Source: CAD feature listing. Evaluate the final solid. Frame: model axes, mm. A direction names the side the tool comes from. Round coordinates to 2 decimals unless told otherwise and drop trailing zeros. Write each loop counter-clockwise with the first axis right and the second up, starting at its lowest first coordinate (ties: lowest second). Pieces come first, ordered by that corner, then holes. Notation, with made-up numbers: M -21.5,50.5 L 32.5,50.5 A15 cw 32.5,74.5 Z; hole C 37,89.25 d4. An arc over 180 degrees is marked long. Use a Markdown table: item, result.
```python
from build123d import *

# Parameters (mm, degrees)
EXTRUDE_1_DEPTH          = 4
EXTRUDE_2_DEPTH          = 9
CHAMFER_1_SIZE           = 1
CHAMFER_2_SIZE           = 1
CHAMFER_3_SIZE           = 1
CHAMFER_4_SIZE           = 1
CUT_EXTRUDE_1_DEPTH      = 24.216373532
CUT_EXTRUDE_1_DEPTH_BACK = 24.216373532
SKETCH_4_R               = 2
CHAMFER_5_SIZE           = 1


with BuildPart() as part:
    # 草图1 → 凸台-拉伸1 (new body)
    with BuildSketch(Plane.XY):
        Polygon((15, -3), (15, 3), (5, 5), (-5, 5), (-15, 3), (-15, -3), (-5, -5), (5, -5), align=None)
    extrude_1 = extrude(amount=EXTRUDE_1_DEPTH)

    # 草图2 → 凸台-拉伸2 (add)
    with BuildSketch(Plane(origin=(0, 0, 0), x_dir=(-1, 0, 0), z_dir=(0, 0, -1))):
        Polygon((0, 5), (-3.535533906, 3.535533906), (-5, 0), (-3.535533906, -3.535533906), (0, -5), (3.535533906, -3.535533906), (5, 0), (3.535533906, 3.535533906), align=None)
    extrude(amount=EXTRUDE_2_DEPTH)

    # 镜向1: 凸台-拉伸1 across plane
    add(extrude_1.mirror(Plane(origin=(0, 0, -4.5), x_dir=(1, 0, 0), z_dir=(0, 0, -1))))

    # 倒角1
    # the kernel refuses this chamfer: 1 mm, written as the material it takes off along each edge
    with BuildSketch(Plane(origin=(-17.521742642, -2.495651472, 0), x_dir=(0.19611613513818427, 0.9805806756909201, 0), z_dir=(0.9805806756909201, -0.19611613513818427, 0))) as chamfer_1_piece_1_section:
        Polygon((CHAMFER_1_SIZE, 0), (0, CHAMFER_1_SIZE), (0, 0), align=None)
    chamfer_1_piece_1 = extrude(amount=20.484770979, mode=Mode.PRIVATE)
    chamfer_1_piece_1 = split(chamfer_1_piece_1, bisect_by=Plane(origin=(-15.841163755, 1.561624871, 0), z_dir=(-0.3826834323650901, -0.9238795325112866, 0)), keep=Keep.TOP, mode=Mode.PRIVATE)
    add(chamfer_1_piece_1, mode=Mode.SUBTRACT)
    with BuildSketch(Plane(origin=(-15, 5.571682988, 0), x_dir=(1, 0, 0), z_dir=(0, -1, 0))) as chamfer_1_piece_2:
        Polygon((CHAMFER_1_SIZE, 0), (0, CHAMFER_1_SIZE), (0, 0), align=None)
    extrude(amount=11.143365976, mode=Mode.SUBTRACT)
    with BuildSketch(Plane(origin=(2.565227926, 6.513045585, 0), x_dir=(0.1961161351381843, -0.9805806756909201, 0), z_dir=(-0.9805806756909201, -0.19611613513818427, 0))) as chamfer_1_piece_3_section:
        Polygon((CHAMFER_1_SIZE, 0), (0, CHAMFER_1_SIZE), (0, 0), align=None)
    chamfer_1_piece_3 = extrude(amount=20.484770979, mode=Mode.PRIVATE)
    chamfer_1_piece_3 = split(chamfer_1_piece_3, bisect_by=Plane(origin=(2.724501391, 6.128525427, 0), z_dir=(-0.38268343236508795, 0.9238795325112875, 0)), keep=Keep.TOP, mode=Mode.PRIVATE)
    add(chamfer_1_piece_3, mode=Mode.SUBTRACT)

    # 倒角2
    # the kernel refuses this chamfer: 1 mm, written as the material it takes off along each edge
    with BuildSketch(Plane(origin=(-2.565227926, -6.513045585, 0), x_dir=(-0.1961161351381843, 0.9805806756909202, 0), z_dir=(0.9805806756909201, 0.19611613513818427, 0))) as chamfer_2_piece_1_section:
        Polygon((CHAMFER_2_SIZE, 0), (0, CHAMFER_2_SIZE), (0, 0), align=None)
    chamfer_2_piece_1 = extrude(amount=20.484770979, mode=Mode.PRIVATE)
    chamfer_2_piece_1 = split(chamfer_2_piece_1, bisect_by=Plane(origin=(-2.724501391, -6.128525427, 0), z_dir=(0.3826834323650899, -0.9238795325112867, 0)), keep=Keep.TOP, mode=Mode.PRIVATE)
    add(chamfer_2_piece_1, mode=Mode.SUBTRACT)
    with BuildSketch(Plane(origin=(15, -5.571682988, 0), x_dir=(-1, 0, 0), z_dir=(0, 1, 0))) as chamfer_2_piece_2:
        Polygon((CHAMFER_2_SIZE, 0), (0, CHAMFER_2_SIZE), (0, 0), align=None)
    extrude(amount=11.143365976, mode=Mode.SUBTRACT)
    with BuildSketch(Plane(origin=(17.521742642, 2.495651472, 0), x_dir=(-0.19611613513818427, -0.9805806756909201, 0), z_dir=(-0.9805806756909201, 0.19611613513818427, 0))) as chamfer_2_piece_3_section:
        Polygon((CHAMFER_2_SIZE, 0), (0, CHAMFER_2_SIZE), (0, 0), align=None)
    chamfer_2_piece_3 = extrude(amount=20.484770979, mode=Mode.PRIVATE)
    chamfer_2_piece_3 = split(chamfer_2_piece_3, bisect_by=Plane(origin=(15.841163755, -1.561624871, 0), z_dir=(0.38268343236509167, 0.923879532511286, 0)), keep=Keep.TOP, mode=Mode.PRIVATE)
    add(chamfer_2_piece_3, mode=Mode.SUBTRACT)

    # 倒角3
    # the kernel refuses this chamfer: 1 mm, written as the material it takes off along each edge
    with BuildSketch(Plane(origin=(-17.521742642, -2.495651472, -9), x_dir=(0.19611613513818427, 0.9805806756909201, 0), z_dir=(0.9805806756909201, -0.19611613513818427, 0))) as chamfer_3_piece_1_section:
        Polygon((CHAMFER_3_SIZE, 0), (0, -CHAMFER_3_SIZE), (0, 0), align=None)
    chamfer_3_piece_1 = extrude(amount=20.484770979, mode=Mode.PRIVATE)
    chamfer_3_piece_1 = split(chamfer_3_piece_1, bisect_by=Plane(origin=(-15.841163755, 1.561624871, -9), z_dir=(-0.3826834323650901, -0.9238795325112866, 0)), keep=Keep.TOP, mode=Mode.PRIVATE)
    add(chamfer_3_piece_1, mode=Mode.SUBTRACT)
    with BuildSketch(Plane(origin=(-15, 5.571682988, -9), x_dir=(1, 0, 0), z_dir=(0, -1, 0))) as chamfer_3_piece_2:
        Polygon((CHAMFER_3_SIZE, 0), (0, -CHAMFER_3_SIZE), (0, 0), align=None)
    extrude(amount=11.143365976, mode=Mode.SUBTRACT)
    with BuildSketch(Plane(origin=(2.565227926, 6.513045585, -9), x_dir=(0.1961161351381843, -0.9805806756909202, 0), z_dir=(-0.9805806756909201, -0.19611613513818427, 0))) as chamfer_3_piece_3_section:
        Polygon((CHAMFER_3_SIZE, 0), (0, -CHAMFER_3_SIZE), (0, 0), align=None)
    chamfer_3_piece_3 = extrude(amount=20.484770979, mode=Mode.PRIVATE)
    chamfer_3_piece_3 = split(chamfer_3_piece_3, bisect_by=Plane(origin=(2.724501391, 6.128525427, -9), z_dir=(-0.38268343236508795, 0.9238795325112875, 0)), keep=Keep.TOP, mode=Mode.PRIVATE)
    add(chamfer_3_piece_3, mode=Mode.SUBTRACT)

    # 倒角4
    # the kernel refuses this chamfer: 1 mm, written as the material it takes off along each edge
    with BuildSketch(Plane(origin=(-2.565227926, -6.513045585, -9), x_dir=(0, 0, -1), z_dir=(0.9805806756909201, 0.19611613513818427, 0))) as chamfer_4_piece_1_section:
        Polygon((CHAMFER_4_SIZE, 0), (0, CHAMFER_4_SIZE), (0, 0), align=None)
    chamfer_4_piece_1 = extrude(amount=20.484770979, mode=Mode.PRIVATE)
    chamfer_4_piece_1 = split(chamfer_4_piece_1, bisect_by=Plane(origin=(-2.724501391, -6.128525427, -9), z_dir=(0.3826834323650899, -0.9238795325112867, 0)), keep=Keep.TOP, mode=Mode.PRIVATE)
    add(chamfer_4_piece_1, mode=Mode.SUBTRACT)
    with BuildSketch(Plane(origin=(15, -5.571682988, -9), x_dir=(0, 0, -1), z_dir=(0, 1, 0))) as chamfer_4_piece_2:
        Polygon((CHAMFER_4_SIZE, 0), (0, CHAMFER_4_SIZE), (0, 0), align=None)
    extrude(amount=11.143365976, mode=Mode.SUBTRACT)
    with BuildSketch(Plane(origin=(17.521742642, 2.495651472, -9), x_dir=(0, 0, -1), z_dir=(-0.9805806756909201, 0.19611613513818427, 0))) as chamfer_4_piece_3_section:
        Polygon((CHAMFER_4_SIZE, 0), (0, CHAMFER_4_SIZE), (0, 0), align=None)
    chamfer_4_piece_3 = extrude(amount=20.484770979, mode=Mode.PRIVATE)
    chamfer_4_piece_3 = split(chamfer_4_piece_3, bisect_by=Plane(origin=(15.841163755, -1.561624871, -9), z_dir=(0.38268343236509167, 0.923879532511286, 0)), keep=Keep.TOP, mode=Mode.PRIVATE)
    add(chamfer_4_piece_3, mode=Mode.SUBTRACT)

    # 草图4 → 切除-拉伸1 (cut, two sides: drawn at the far end of the back side and taken through both)
    with BuildSketch(Plane(origin=(0, 0, -13), x_dir=(-1, 0, 0), z_dir=(0, 0, -1)).offset(-CUT_EXTRUDE_1_DEPTH_BACK)):
        Circle(SKETCH_4_R)
        with Locations((10, 0)):
            Circle(SKETCH_4_R)
        with Locations(Location((-10, 0, 0), (0, 0, 180))):
            Circle(SKETCH_4_R)
    extrude(amount=CUT_EXTRUDE_1_DEPTH + CUT_EXTRUDE_1_DEPTH_BACK, mode=Mode.SUBTRACT)

    # 倒角5
    # the kernel refuses this chamfer: 1 mm, written as the material it takes off along each edge
    with BuildSketch(Plane(origin=(10, 0, 0), x_dir=(1, 0, 0), z_dir=(0, 1, 0))) as chamfer_5_piece_1:
        Polygon((2 + CHAMFER_5_SIZE, 0), (2, -CHAMFER_5_SIZE), (2, 0), align=None)
    revolve(axis=Axis((10, 0, 0), (0, 0, -1)), mode=Mode.SUBTRACT)
    with BuildSketch(Plane(origin=(10, 0, -9), x_dir=(1, 0, 0), z_dir=(0, 1, 0))) as chamfer_5_piece_2:
        Polygon((2 + CHAMFER_5_SIZE, 0), (2, CHAMFER_5_SIZE), (2, 0), align=None)
    revolve(axis=Axis((10, 0, -9), (0, 0, -1)), mode=Mode.SUBTRACT)
    with BuildSketch(Plane(origin=(-10, 0, -9), x_dir=(-1, 0, 0), z_dir=(0, -1, 0))) as chamfer_5_piece_3:
        Polygon((2, CHAMFER_5_SIZE), (2 + CHAMFER_5_SIZE, 0), (2, 0), align=None)
    revolve(axis=Axis((-10, 0, -9), (0, 0, -1)), mode=Mode.SUBTRACT)
    with BuildSketch(Plane(origin=(-10, 0, 0), x_dir=(-1, 0, 0), z_dir=(0, -1, 0))) as chamfer_5_piece_4:
        Polygon((2, -CHAMFER_5_SIZE), (2 + CHAMFER_5_SIZE, 0), (2, 0), align=None)
    revolve(axis=Axis((-10, 0, 0), (0, 0, -1)), mode=Mode.SUBTRACT)


solid = part.part
```
Q1. Line query: L1, parallel to X at y = 0, z = 2.55; L2, parallel to Y at x = 0, z = -5.75. Output: solid intervals per line, ascending.
Results are:
| item | result |
|---|---|
| L1 | -15 to -12, -8 to -2, 2 to 8, 12 to 15 |
| L2 | -5 to -2, 2 to 5 |
Q2. Section B-B on z = -4.25. Return loops of the section in (x, y), plus the area to 3 significant figures.
Results are:
| item | result |
|---|---|
| outline | M -5,0 L -3.54,-3.54 L 0,-5 L 3.54,-3.54 L 5,0 L 3.54,3.54 L 0,5 L -3.54,3.54 Z; hole C 0,0 d4 |
| area | 58.1 mm^2 |
Q3. First-contact query: pin 1 Ø8 at (x, z) = (-6, -1.5) entering from +Y. Flat tip, straight axial feed; report the tip coordinate or a pass-through.
Results are:
| item | result |
|---|---|
| pin 1 | y = 5 |
Q4. Section C-C on y = 4.25. Return loops of the section in (x, z).
Results are:
| item | result |
|---|---|
| outline | M -8.75,-13 L 8.75,-13 L 8.75,-10 L 3.65,-9 L 1.81,-9 L 1.81,0 L 3.65,0 L 8.75,1 L 8.75,4 L -8.75,4 L -8.75,1 L -3.65,0 L -1.81,0 L -1.81,-9 L -3.65,-9 L -8.75,-10 Z |
Q5. Mould query, pull axis Y, two halves, no side actions, for faces 5 (the cylindrical face through (8.4, 1.2, -11.5)), 6 (the cylindrical face through (8.4, 1.2, 2.5)), 7 (the flat face through (-9.038, 3.675, 0.493)), 8 (the flat face through (-14.5, 0, 0.5)). Classes: +Y half, -Y half, draft (parallel to the pull), parting line (faces both ways), or undercut.
Results are:
| item | result |
|---|---|
| face 5 | undercut |
| face 6 | undercut |
| face 7 | +Y half |
| face 8 | draft |
Q6. Section D-D on y = 1.5. Give the number of separate pieces and of enclosed holes in the cut face, plus the area to 3 significant figures.
Results are:
| item | result |
|---|---|
| separate pieces | 6 |
| enclosed holes | 0 |
| area | 224 mm^2 |
Q7. Section A-A on z = -11.75. Return loops of the section in (x, y), plus the area to 3 significant figures.
Results are:
| item | result |
|---|---|
| outline | M -15,-3 L -5,-5 L 5,-5 L 15,-3 L 15,3 L 5,5 L -5,5 L -15,3 Z; hole C -10,0 d4; hole C 0,0 d4; hole C 10,0 d4 |
| area | 222 mm^2 |
Q8. Reachability of faces 1 (the flat face through (9.25, 3.63, 0.49)), 2 (the flat face through (-6, 0, 0)), 3 (the flat face through (5.3, 0, -9)), 4 (the flat face through (13.2, 0, -9)) from +Z, -Z, +X, -X, +Y, -Y: full face, straight path, thin tool, end or side. Return the list, or none.
Results are:
| item | result |
|---|---|
| face 1 | +X, +Y |
| face 2 | -X |
| face 3 | +X |
| face 4 | +X, +Y, -Y |
